Build history of the part. All positions in model axes, mm. A direction names the side the tool comes from. Round coordinates to 2 decimals unless told otherwise and drop trailing zeros. Order: outer loops, then holes, each group sorted by start corner. A loop starts at its lowest first (then second) coordinate and runs counter-clockwise, first axis right, second up. Notation, with made-up numbers: M -8.5,52.5 L 2.5,52.5 A37 ccw 2.5,91.5 Z; hole C 32.25,-17 d3. An arc over 180 degrees is marked long. Use CSV: the item, a comma, the result in double quotes.
from build123d import *

# Parameters (mm, degrees)
F0_R     = 77.5
F0_R_2   = 5.125
F0_R_3   = 56
F0_R_4   = 20.5
F0_R_5   = 2.6
F1_DEPTH = 13
F2_DEPTH = 25
F0_R_6   = 17.25
F3_DEPTH = 10
F4_DEPTH = 6
F5_DEPTH = 6


with BuildPart() as f1:
    # F0 (on Top) → F1 (new body)
    with BuildSketch(Plane.XY):
        Circle(F0_R)
        with Locations((-60.621778, -35)):
            Circle(F0_R_2, mode=Mode.SUBTRACT)
        with Locations((60.621778, -35)):
            Circle(F0_R_2, mode=Mode.SUBTRACT)
        Circle(F0_R_3, mode=Mode.SUBTRACT)
        with Locations((0, 70)):
            Circle(F0_R_2, mode=Mode.SUBTRACT)
        Circle(F0_R_3)
        Polygon((-4.6, -43), (-2.3, -39.016283), (2.3, -39.016283), (4.6, -43), (2.3, -46.983717), (-2.3, -46.983717), align=None, mode=Mode.SUBTRACT)
        Polygon((-34.939092, 25.483717), (-32.639092, 21.5), (-34.939092, 17.516283), (-39.539092, 17.516283), (-41.839092, 21.5), (-39.539092, 25.483717), align=None, mode=Mode.SUBTRACT)
        Circle(F0_R_4, mode=Mode.SUBTRACT)
        Polygon((34.939092, 17.516283), (32.639092, 21.5), (34.939092, 25.483717), (39.539092, 25.483717), (41.839092, 21.5), (39.539092, 17.516283), align=None, mode=Mode.SUBTRACT)
        with Locations((0, 70)):
            Circle(F0_R_2)
        with Locations((0, 70)):
            Circle(F0_R_5, mode=Mode.SUBTRACT)
        Polygon((-34.939092, 17.516283), (-32.639092, 21.5), (-34.939092, 25.483717), (-39.539092, 25.483717), (-41.839092, 21.5), (-39.539092, 17.516283), align=None)
        with Locations((-37.239092, 21.5)):
            Circle(F0_R_5, mode=Mode.SUBTRACT)
        Polygon((34.939092, 25.483717), (32.639092, 21.5), (34.939092, 17.516283), (39.539092, 17.516283), (41.839092, 21.5), (39.539092, 25.483717), align=None)
        with Locations((37.239092, 21.5)):
            Circle(F0_R_5, mode=Mode.SUBTRACT)
        with Locations((60.621778, -35)):
            Circle(F0_R_2)
        with Locations((60.621778, -35)):
            Circle(F0_R_5, mode=Mode.SUBTRACT)
        Polygon((2.3, -39.016283), (-2.3, -39.016283), (-4.6, -43), (-2.3, -46.983717), (2.3, -46.983717), (4.6, -43), align=None)
        with Locations((0, -43)):
            Circle(F0_R_5, mode=Mode.SUBTRACT)
        with Locations((-60.621778, -35)):
            Circle(F0_R_2)
        with Locations((-60.621778, -35)):
            Circle(F0_R_5, mode=Mode.SUBTRACT)
    extrude(amount=F1_DEPTH)

    # F0 (on Top) → F2 (join)
    with BuildSketch(Plane.XY):
        Circle(F0_R)
        with Locations((-60.621778, -35)):
            Circle(F0_R_2, mode=Mode.SUBTRACT)
        with Locations((60.621778, -35)):
            Circle(F0_R_2, mode=Mode.SUBTRACT)
        Circle(F0_R_3, mode=Mode.SUBTRACT)
        with Locations((0, 70)):
            Circle(F0_R_2, mode=Mode.SUBTRACT)
        with Locations((0, 70)):
            Circle(F0_R_2)
        with Locations((0, 70)):
            Circle(F0_R_5, mode=Mode.SUBTRACT)
        with Locations((60.621778, -35)):
            Circle(F0_R_2)
        with Locations((60.621778, -35)):
            Circle(F0_R_5, mode=Mode.SUBTRACT)
        with Locations((-60.621778, -35)):
            Circle(F0_R_2)
        with Locations((-60.621778, -35)):
            Circle(F0_R_5, mode=Mode.SUBTRACT)
    extrude(amount=F2_DEPTH)

    # F0 (on Top) → F3 (join)
    with BuildSketch(Plane.XY):
        Circle(F0_R_4)
        Circle(F0_R_6, mode=Mode.SUBTRACT)
    extrude(amount=F3_DEPTH)

    # F0 (on Top) → F4 (cut)
    with BuildSketch(Plane.XY):
        with Locations((0, 70)):
            Circle(F0_R_2)
        with Locations((0, 70)):
            Circle(F0_R_5, mode=Mode.SUBTRACT)
        with Locations((-60.621778, -35)):
            Circle(F0_R_2)
        with Locations((-60.621778, -35)):
            Circle(F0_R_5, mode=Mode.SUBTRACT)
        with Locations((60.621778, -35)):
            Circle(F0_R_2)
        with Locations((60.621778, -35)):
            Circle(F0_R_5, mode=Mode.SUBTRACT)
    extrude(amount=F4_DEPTH, mode=Mode.SUBTRACT)

    # F0 (on Top) → F5 (cut)
    with BuildSketch(Plane.XY):
        Polygon((34.939092, 25.483717), (32.639092, 21.5), (34.939092, 17.516283), (39.539092, 17.516283), (41.839092, 21.5), (39.539092, 25.483717), align=None)
        with Locations((37.239092, 21.5)):
            Circle(F0_R_5, mode=Mode.SUBTRACT)
        Polygon((-34.939092, 17.516283), (-32.639092, 21.5), (-34.939092, 25.483717), (-39.539092, 25.483717), (-41.839092, 21.5), (-39.539092, 17.516283), align=None)
        with Locations((-37.239092, 21.5)):
            Circle(F0_R_5, mode=Mode.SUBTRACT)
        Polygon((2.3, -39.016283), (-2.3, -39.016283), (-4.6, -43), (-2.3, -46.983717), (2.3, -46.983717), (4.6, -43), align=None)
        with Locations((0, -43)):
            Circle(F0_R_5, mode=Mode.SUBTRACT)
    extrude(amount=F5_DEPTH, mode=Mode.SUBTRACT)


solid = f1.part
(1) Two-plate mould, pull along Y, no slides. Class faces 4 (the face through (40.705, 23.464, 2.958)), 5 (the face through (-16.8, -75.657, 12.325)): released by +Y, released by -Y, zero draft, split by the parting line, or undercut.
Answer block:
face 4,"undercut"
face 5,"split by the parting line"
(2) Cut at C-C, the plane y = 70. Give the cut face in (x, z) (3 decimals), and give its area (3 significant figures).
Answer block:
outline,"M -33.26,0 L -5.125,0 L -5.125,6 L -2.6,6 L -2.6,25 L -33.26,25 Z; M 2.6,6 L 5.125,6 L 5.125,0 L 33.26,0 L 33.26,25 L 2.6,25 Z"
area,"1,500 mm²"
(3) Cut at D-D, the plane y = -35. Give the cut face in (x, z), and give its area (3 significant figures).
Answer block:
outline,"M -69.15,0 L -65.75,0 L -65.75,6 L -63.22,6 L -63.22,25 L -69.15,25 Z; M -58.02,6 L -55.5,6 L -55.5,0 L 55.5,0 L 55.5,6 L 58.02,6 L 58.02,25 L 43.71,25 L 43.71,13 L -43.71,13 L -43.71,25 L -58.02,25 Z; M 63.22,6 L 65.75,6 L 65.75,0 L 69.15,0 L 69.15,25 L 63.22,25 Z"
area,"2,090 mm²"
(4) Cut at B-B, the plane z = 17.25. Give the cut face in (x, y).
Answer block:
outline,"C 0,0 d155; hole C -60.62,-35 d5.2; hole C 0,0 d112; hole C 0,70 d5.2; hole C 60.62,-35 d5.2"
(5) Tool access for faces 1 (the face through (-4.444, -20.013, 11.479)), 2 (the face through (16.453, 5.181, 4.93)), 3 (the face through (-64.69, -38.12, 2.96)): list every direction of +Z, -Z, +X, -X, +Y, -Y with a clear straight run to the whole face (end or side of a thin tool).
Answer block:
face 1,"+Z"
face 2,"+Z, -Z"
face 3,"-Z"
(6) Drop flat-ended pins along their axis: pin 1 (3 mm diameter, centred on x = 41, y = 14, fed in from +Z); pin 2 (5 mm diameter, centred on x = -20.5, z = 15, fed in from -Y); pin 3 (8 mm diameter, centred on x = -49, y = 19.5, fed in from +Z); pin 4 (9 mm diameter, centred on x = 0, y = 70, fed in from -Z). Give the stop position or say it passes through.
Answer block:
pin 1,"stops at z = 13"
pin 2,"stops at y = -75.38"
pin 3,"stops at z = 25"
pin 4,"stops at z = 6"
(7) Wall check: line 1 (Y direction, x = 0, z = 3.05) (3 decimals); line 2 (Z direction, x = -12.5, y = -17); line 3 (Y direction, x = -28.5, z = 22.25). Give the ranges that are in metal, low to high. Write a range as from..to.
Answer block:
line 1,"y = -77.5..-46.984, -39.016..-17.25, 17.25..64.875, 75.125..77.5"
line 2,"z = 0..13"
line 3,"y = -72.07..-48.21, 48.21..72.07"
(8) Cut at A-A, the plane x = 0. Count the separate pieces of the cut face and the enclosed holes in it, and give its area (3 significant figures).
Answer block:
separate pieces,"4"
enclosed holes,"0"
area,"1,820 mm²"
